```python
from build123d import *

# Parameters (mm, degrees)
SKETCH1_R           = 60
BOSS_EXTRUDE1_DEPTH = 35
SKETCH2_R           = 20.1
CUT_EXTRUDE1_DEPTH  = 17
SKETCH3_R           = 3
CUT_EXTRUDE2_DEPTH  = 10
SKETCH5_R           = 50
CUT_EXTRUDE3_DEPTH  = 10
MOVE_FACE1_BY       = 20
MOVE_FACE4_BY       = 10
SKETCH6_R           = 2.5
CUT_EXTRUDE4_DEPTH  = 102.118742081
CIRPATTERN1_COUNT   = 2
CIRPATTERN1_ANGLE   = 90


with BuildPart() as part:
    # Sketch1 → Boss-Extrude1 (new body)
    with BuildSketch(Plane(origin=(0, 0, 0), x_dir=(1, 0, 0), z_dir=(0, 1, 0))):
        with Locations(Location((0, 0, 0), (0, 0, 270))):
            Circle(SKETCH1_R)
    extrude(amount=BOSS_EXTRUDE1_DEPTH)

    # Sketch2 → Cut-Extrude1 (cut)
    with BuildSketch(Plane(origin=(0, 35, 0), x_dir=(1, 0, 0), z_dir=(0, 1, 0))):
        with Locations(Location((0, 0, 0), (0, 0, 270))):
            Circle(SKETCH2_R)
    extrude(amount=-CUT_EXTRUDE1_DEPTH, mode=Mode.SUBTRACT)

    # Sketch3 → Cut-Extrude2 (cut)
    with BuildSketch(Plane.XZ):
        with Locations(Location((-30, 30, 0), (0, 0, 270))):
            Circle(SKETCH3_R)
        with Locations(Location((30, 30, 0), (0, 0, 270))):
            Circle(SKETCH3_R)
        with Locations(Location((30, -30, 0), (0, 0, 270))):
            Circle(SKETCH3_R)
        with Locations(Location((-30, -30, 0), (0, 0, 270))):
            Circle(SKETCH3_R)
    extrude(amount=-CUT_EXTRUDE2_DEPTH, mode=Mode.SUBTRACT)

    # Sketch5 → Cut-Extrude3 (cut)
    with BuildSketch(Plane(origin=(0, 35, 0), x_dir=(1, 0, 0), z_dir=(0, 1, 0))):
        with Locations(Location((0, 0, 0), (0, 0, 270))):
            Circle(SKETCH5_R)
    extrude(amount=-CUT_EXTRUDE3_DEPTH, mode=Mode.SUBTRACT)

    # Move Face1: a face moved outward by 20.0
    extrude(part.faces().sort_by_distance((-30, 35, 48))[0], amount=MOVE_FACE1_BY, dir=(0, 1, 0))

    # Move Face4: a face moved inward by 10.0
    extrude(part.faces().sort_by_distance((0, 18, 0))[0], amount=MOVE_FACE4_BY, dir=(0, -1, 0), mode=Mode.SUBTRACT)

    # Sketch6 → Cut-Extrude4 (cut, symmetric)
    with BuildSketch(Plane(origin=(0, 0, 0), x_dir=(0, 0, -1), z_dir=(1, 0, 0))):
        with Locations((0, 40)):
            Circle(SKETCH6_R)
    cut_extrude4 = extrude(amount=CUT_EXTRUDE4_DEPTH, both=True, mode=Mode.SUBTRACT)

    # CirPattern1: Cut-Extrude4 ×2 about axis
    cirpattern1_axis = Axis((0, 35, 0), (0, -1, 0))
    for i in range(1, CIRPATTERN1_COUNT):
        add(cut_extrude4.rotate(cirpattern1_axis, i * CIRPATTERN1_ANGLE / (CIRPATTERN1_COUNT - 1)), mode=Mode.SUBTRACT)


solid = part.part
```
CAD build for the part. Positions are in the model's coordinates, mm. A direction names the side the tool comes from. Round coordinates to 2 decimals unless told otherwise and drop trailing zeros. Write each loop counter-clockwise with the first axis right and the second up, starting at its lowest first coordinate (ties: lowest second). Pieces come first, ordered by that corner, then holes.
Item 1: Band-saw the part on A-A on z = 0. Write the cut outline in (x, y).
Filled in:
outline: (-60, 0) - (60, 0) - (60, 37.5) - (50, 37.5) - (50, 25) - (20.1, 25) - (20.1, 8) - (-20.1, 8) - (-20.1, 25) - (-50, 25) - (-50, 37.5) - (-60, 37.5) - close; (-60, 42.5) - (-50, 42.5) - (-50, 55) - (-60, 55) - close; (50, 42.5) - (60, 42.5) - (60, 55) - (50, 55) - close
Item 2: Band-saw the part on D-D on x = 30. Write the cut outline in (y, z).
Filled in:
outline: (0, -51.96) - (55, -51.96) - (55, -40) - (25, -40) - (25, 40) - (55, 40) - (55, 51.96) - (0, 51.96) - (0, 33) - (10, 33) - (10, 27) - (0, 27) - (0, -27) - (10, -27) - (10, -33) - (0, -33) - close
Item 3: Mould opens along Z. For faces 4 (the flat face through (45, 55, -23)), 5 (the cylindrical face through (2.64, 27.12, -59.94)), 6 (the cylindrical face through (-54.9, 37.56, 0.54)) say: released by +Z, released by -Z, zero draft, split by the parting line, or undercut.
Filled in:
face 4: zero draft
face 5: split by the parting line
face 6: undercut
Item 4: Tool access for faces 1 (the cylindrical face through (55.04, 37.56, 0.54)), 2 (the cylindrical face through (0.88, 16.62, -20.08)), 3 (the flat face through (-30, 10, 30)): list every direction of +Z, -Z, +X, -X, +Y, -Y with a clear straight run to the whole face (end or side of a thin tool).
Filled in:
face 1: +X, -X
face 2: +Y
face 3: -Y
Item 5: Drop flat-ended pins along their axis: pin 1 Ø1.5 at (x, y) = (-30.5, 37) entering from -Z; pin 2 Ø1.5 at (x, y) = (-26, 49.5) entering from -Z; pin 3 Ø3.5 at (x, z) = (30, 30) entering from -Y. Give the stop position or say it passes through.
Filled in:
pin 1: stops at z = -52.11
pin 2: stops at z = -54.43
pin 3: stops at y = 10
Item 6: Drill centre lines: L1, parallel to X at y = 16, z = 0; L2, parallel to Y at x = 11, z = 7.5; L3, parallel to Z at x = -7, y = 38. Where is each one in solid material? Low to high.
Filled in:
L1: x = -60 to -20.1, 20.1 to 60
L2: y = 0 to 8
L3: z = -59.59 to -49.51, 49.51 to 59.59
Item 7: Band-saw the part on B-B on y = 40. Write the cut outline in (x, z).
Filled in:
outline: (-59.95, -2.5) arc R60 ccw to (-2.5, -59.95) - (-2.5, -49.94) arc R50 cw to (-49.94, -2.5) - close; (-59.95, 2.5) - (-49.94, 2.5) arc R50 cw to (-2.5, 49.94) - (-2.5, 59.95) arc R60 ccw to start; (2.5, -59.95) arc R60 ccw to (59.95, -2.5) - (49.94, -2.5) arc R50 cw to (2.5, -49.94) - close; (2.5, 49.94) arc R50 cw to (49.94, 2.5) - (59.95, 2.5) arc R60 ccw to (2.5, 59.95) - close
Item 8: Band-saw the part on C-C on y = 51.5. Write the cut outline in (x, z), then the cut area to 3 significant figures.
Filled in:
outline: circle Ø120 at (0, 0); hole circle Ø100 at (0, 0)
area: 3,460 mm2
